Print and shaded views of the part. All mm, measured from the part's lowest x, y and z. Give positions to 0.01 mm unless a question says otherwise; leave off trailing zeros. Write each loop counter-clockwise with the first axis right and the second up, starting at its lowest first coordinate (ties: lowest second). Pieces come first, ordered by that corner, then holes. Notation, with made-up numbers: (85, 57.5) - (126, 57.5) arc R20 cw to (126, 63.5) - close; hole circle Ø3 at (0.5, -32.75). An arc over 180 degrees is marked (long way). Use one line per item in the form item = value. Start each with the question number.
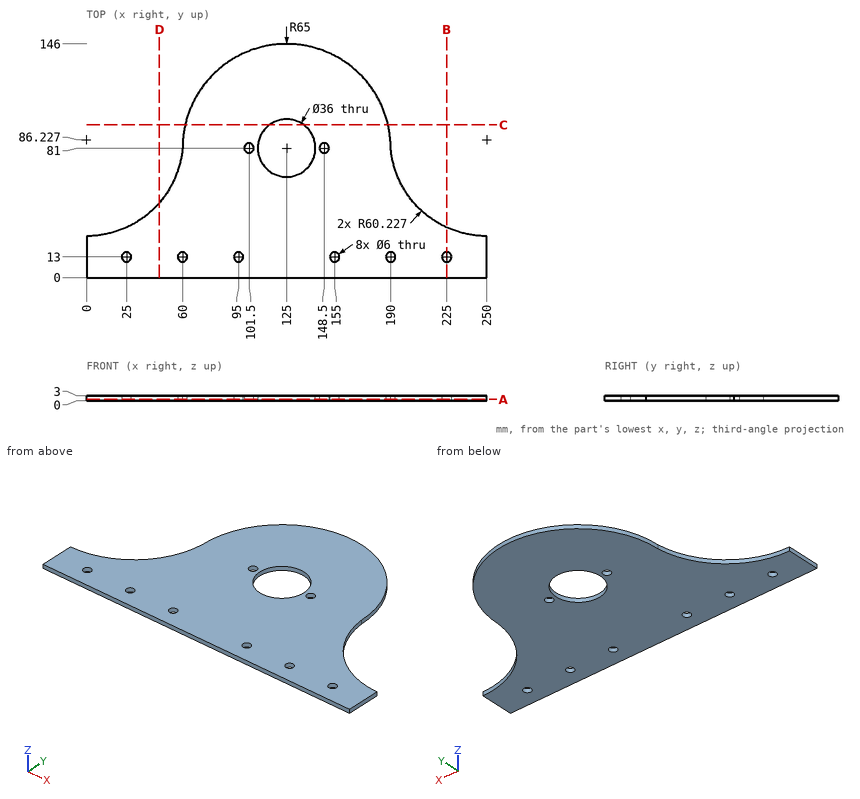
(1) Cut at A-A, the plane z = 0.7. State how many separate pieces and enclosed holes the cut face has, then the cut area to 3 significant figures.
(2) Cut at D-D, the plane x = 45.5. Give the cut face in (y, z), then the cut area to 3 significant figures.
(3) Wall check: line 1 (Y direction, x = 116.5, z = 0.9); line 2 (Y direction, x = 138, z = 2.5); line 3 (X direction, y = 72, z = 1.8). Give the ranges that are in metal, low to high. Write a range as from..to.
(4) Cut at C-C, the plane y = 95.5. Give the cut face in (x, z) (1 decimal).
(5) Cut at B-B, the plane x = 225. Give the cut face in (y, z).
Solution:
q1.separate_pieces = 1
q1.enclosed_holes = 9
q1.area = 20,600 mm2
q2.outline = (0, 0) - (46.77, 0) - (46.77, 3) - (0, 3) - close
q2.area = 140 mm2
q3.line_1 = 0..65.13, 96.87..145.44
q3.line_2 = 0..68.55, 93.45..144.69
q3.line_3 = 58.52..109.41, 140.59..191.48
q4.outline = (61.6, 0) - (114.3, 0) - (114.3, 3) - (61.6, 3) - close; (135.7, 0) - (188.4, 0) - (188.4, 3) - (135.7, 3) - close
q5.outline = (0, 0) - (10, 0) - (10, 3) - (0, 3) - close; (16, 0) - (31.43, 0) - (31.43, 3) - (16, 3) - close
